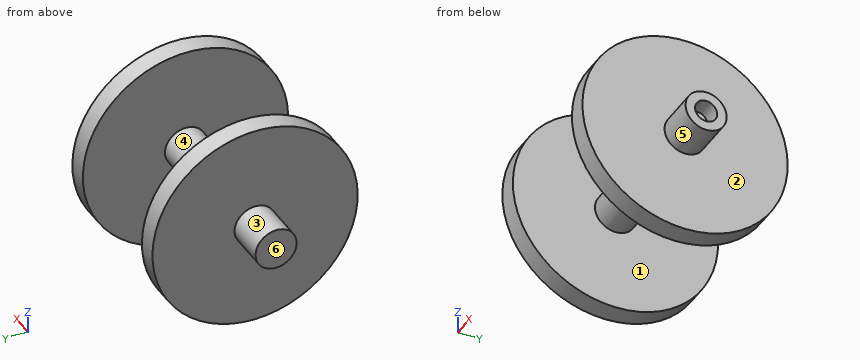
```python
from build123d import *

# Parameters (mm, degrees)
SKETCH4_R          = 3.429
CUT_EXTRUDE1_DEPTH = 5.715


with BuildPart() as part:
    # Sketch2 → Revolve1 (revolve)
    with BuildSketch(Plane.XY, mode=Mode.PRIVATE) as revolve1_sk:
        Polygon((0, 31.75), (6.35, 31.75), (6.35, 6.35), (41.91, 6.35), (41.91, 31.75), (48.26, 31.75), (48.26, 6.35), (60.96, 6.35), (60.96, 0), (48.26, 0), (0, 0), (-12.7, 0), (-12.7, 6.35), (0, 6.35), align=None)
    revolve(revolve1_sk.sketch.rotate(Axis((48.26, 0, 0), (-1, 0, 0)), 90), axis=Axis((48.26, 0, 0), (-1, 0, 0)))

    # Sketch4 → Cut-Extrude1 (cut)
    with BuildSketch(Plane(origin=(60.96, 0, 0), x_dir=(0, 0, -1), z_dir=(1, 0, 0))):
        Circle(SKETCH4_R)
    extrude(amount=-CUT_EXTRUDE1_DEPTH, mode=Mode.SUBTRACT)


solid = part.part
```
Can you work these out from the model? Positions are in its coordinate system, mm. Face numbers are marked on the shaded views. A direction names the side the tool comes from. Coordinates: 2 decimals unless noted, no trailing zeros. Order: outer loops, then holes, each group sorted by start corner. A loop starts at its lowest first (then second) coordinate and runs counter-clockwise, first axis right, second up.
1. For the marked faces 4, 5 and 6, which set-ups out of +Z, -Z, +X, -X, +Y, -Y let a thin tool reach every point of the face, with its end or its side?
2. Thinking about a two-plate mould opening in X: for the marked faces 1, 2 and 3, which applies, +X half, -X half, draft (parallel to the pull), parting line (faces both ways), or undercut?
3. If we section it at D-D (z = 0): Please give me the cut outline in (x, y) (3 decimals), then the cut area to 3 significant figures.
4. I'm going to push flat-ended pins straight in: pin 1 (10 mm diameter, centred on y = -15.5, z = 9.5, fed in from +X); pin 2 (19 mm diameter, centred on y = -15.5, z = 3.5, fed in from -X); pin 3 (6 mm diameter, centred on y = 0, z = 0, fed in from +X) (3 decimals); pin 4 (5 mm diameter, centred on x = -4.5, y = -25, fed in from -Z). Where does each tip first touch, or does it pass through?
5. If we section it at C-C (x = 7.5): Please give me the cut outline in (y, z), then the cut area to 3 significant figures.
6. If we section it at A-A (y = 24.5): Please give me the cut outline in (x, z), then the cut area to 3 significant figures.
7. I need wall thicknesses on line 1 (X direction, y = -6, z = 12.5); line 2 (Y direction, x = 56.95, z = 0); line 3 (Y direction, x = 12.5, z = 0). Which ranges of each line are inside material? Lowest first, please.
8. If we section it at B-B (z = -15): Please give me the cut outline in (x, y), then the cut area to 3 significant figures.
Entries:
1. face 4: none
1. face 5: +X
1. face 6: +Z, -Z, -X, +Y, -Y
2. face 1: undercut
2. face 2: +X half
2. face 3: draft
3. outline: (-12.7, -6.35) - (0, -6.35) - (0, -31.75) - (6.35, -31.75) - (6.35, -6.35) - (41.91, -6.35) - (41.91, -31.75) - (48.26, -31.75) - (48.26, -6.35) - (60.96, -6.35) - (60.96, -3.429) - (55.245, -3.429) - (55.245, 3.429) - (60.96, 3.429) - (60.96, 6.35) - (48.26, 6.35) - (48.26, 31.75) - (41.91, 31.75) - (41.91, 6.35) - (6.35, 6.35) - (6.35, 31.75) - (0, 31.75) - (0, 6.35) - (-12.7, 6.35) - close
3. area: 1,540 mm2
4. pin 1: stops at x = 48.26
4. pin 2: stops at x = 0
4. pin 3: stops at x = 55.245
4. pin 4: passes through
5. outline: circle Ø12.7 at (0, 0)
5. area: 127 mm2
6. outline: (0, -20.19) - (6.35, -20.19) - (6.35, 20.19) - (0, 20.19) - close; (41.91, -20.19) - (48.26, -20.19) - (48.26, 20.19) - (41.91, 20.19) - close
6. area: 513 mm2
7. line 1: x = 0 to 6.35, 41.91 to 48.26
7. line 2: y = -6.35 to -3.43, 3.43 to 6.35
7. line 3: y = -6.35 to 6.35
8. outline: (0, -27.98) - (6.35, -27.98) - (6.35, 27.98) - (0, 27.98) - close; (41.91, -27.98) - (48.26, -27.98) - (48.26, 27.98) - (41.91, 27.98) - close
8. area: 711 mm2
